Design review of the part built by this model. Coordinates are the model's own, in mm. A direction names the side the tool comes from. Coordinates: 2 decimals unless noted, no trailing zeros. Write each loop counter-clockwise with the first axis right and the second up, starting at its lowest first coordinate (ties: lowest second). Pieces come first, ordered by that corner, then holes. Notation, with made-up numbers: (77.25, 31.25) -> (103.25, 31.25) arc R15 cw to (103.25, 44.25) -> close; hole circle Ø4 at (61, -4.75). An arc over 180 degrees is marked (long way). Write item = value, one per line. Start each with the question number.
Solid Edge part; units mm, degrees
sketch "Sketch1" plane through (0, 0, 0) normal (0, 0, 1) x (1, 0, 0)
  line L0 (58.55, -37.1) -> (-58.55, -37.1)
  line L1 (-58.55, -37.1) -> (-58.55, 37.1)
  line L2 (-58.55, 37.1) -> (58.55, 37.1)
  line L3 (58.55, 37.1) -> (58.55, -37.1)
extrude "Protrusion1" add sketch "Sketch1" against normal blind 2.5
sketch "Sketch2" plane through (0, 0, 0) normal (0, 0, 1) x (1, 0, 0)
  line L0 (56.55, -35.1) -> (-58.55, -35.1)
  line L1 (-58.55, -35.1) -> (-58.55, -37.1)
  line L2 (-58.55, -37.1) -> (58.55, -37.1)
  line L3 (58.55, -37.1) -> (58.55, 37.1)
  line L4 (58.55, 37.1) -> (-58.55, 37.1)
  line L5 (-58.55, 37.1) -> (-58.55, 35.1)
  line L6 (-58.55, 35.1) -> (56.55, 35.1)
  line L7 (56.55, 35.1) -> (56.55, -35.1)
extrude "ExtrudedProtrusion_2" add sketch "Sketch2" along normal blind 7.5
sketch "Sketch3" plane through (0, 0, -2.5) normal (0, 0, -1) x (-1, 0, 0)
  line L0 (-49.1714, -41.0286) -> (-46.45, -35)
  line L1 (-56.45, -35) -> (-46.45, -35)
  line L2 (-56.45, -35) -> (-53.7286, -41.0286)
  arc A0 (-53.7286, -41.0286) -> (-49.1714, -41.0286) centre (-51.45, -40) ccw
  circle A1 centre (-51.45, -40) radius 1.75
  circle A2 centre (53.55, 40) radius 1.75
  line L3 (58.55, 35) -> (55.8286, 41.0286)
  arc A3 (55.8286, 41.0286) -> (51.2714, 41.0286) centre (53.55, 40) ccw
  line L4 (51.2714, 41.0286) -> (48.55, 35)
  line L5 (48.55, 35) -> (58.55, 35)
extrude "Protrusion2" add sketch "Sketch3" against normal up to vertex (15.5 mm away)
fillet "Round_1" radius 1.5 9 edges at (58.55, -37.1, 2.5) (58.55, 37.1, 2.5) (58.55, 0, -2.5) (4.526, 37.1, -2.5) (-5.576, -37.1, -2.5) (57.026, -37.1, -2.5) (-58.55, 0, -2.5) (-58.55, 37.1, 2.5) (-58.55, -37.1, 2.5)
(1) Mouldability with a two-part tool opening along X and no side actions: class faces 1 (the face through (3, 35.1, 4)), 2 (the face through (51.5, -42.5, 5.1)), 3 (the face through (52, -35, 6)) as pulls with the +X half, pulls with the -X half, needs draft (parallel to the pull), parting line crosses it, or undercut.
(2) For line 1 (Y direction, x = 51.45, z = 6.5); line 2 (Y direction, x = -53.55, z = 3.25); line 3 (Y direction, x = 51.45, z = 8.25), list the stretches that pass through material, from the lowest coordinate up.
(3) For faces 4 (the face through (-5, -35.1, 4)), 5 (the face through (1, 1, -2.5)), 6 (the face through (52.84, -41.06, 5.14)), 7 (the face through (3, 37.1, 3)), 8 (the face through (-56.906, 38.642, 5.142)), list the 3-axis set-ups (+Z, -Z, +X, -X, +Y, -Y) from which the entire face can be reached by the end or side of a thin tool; tool diameter is ignored.
(4) Take a section at B-B, the plane x = -53.55. State the section outline as (y, z) points, then the cut area to 3 significant figures.
(5) Take a section at C-C, the plane x = -18. State the section outline as (y, z) points.
(6) Take a section at D-D, the plane y = 23.5. State the section outline as (x, z) points, then the cut area to 3 significant figures.
(7) Take a section at A-A, the plane z = 11. State the section outline as (x, y) points, then the cut area to 3 significant figures.
(8) For pin 1 Ø1 at (x, z) = (-42.5, 1.5) entering from -Y; pin 2 Ø4 at (x, z) = (-22.5, 4.5) entering from +Y; pin 3 Ø10 at (x, y) = (-43, 1) entering from +Z, all flat-tipped, find the tip position at first contact; note any pin that passes through.
Report:
q1.face_1 = undercut
q1.face_2 = parting line crosses it
q1.face_3 = needs draft
q2.line_1 = -42.5 to -41.75, -38.25 to -35, 35.1 to 37.1
q2.line_2 = -37.1 to -35.1, 35 to 38.25, 41.75 to 42.5
q2.line_3 = -42.5 to -41.75, -38.25 to -35
q3.face_4 = +Z, -X
q3.face_5 = -Z, +X, -X, +Y, -Y
q3.face_6 = +Z, -Z
q3.face_7 = +Z, -Z, +X, +Y
q3.face_8 = +Z, -X, +Y
q4.outline = (-37.1, -1) arc R1.5 ccw to (-35.6, -2.5) -> (38.25, -2.5) -> (38.25, 13) -> (35, 13) -> (35, 0) -> (-35.1, 0) -> (-35.1, 7.5) -> (-37.1, 7.5) -> close; (41.75, -2.5) -> (42.5, -2.5) -> (42.5, 13) -> (41.75, 13) -> close
q4.area = 257 mm2
q5.outline = (-37.1, -1) arc R1.5 ccw to (-35.6, -2.5) -> (35.6, -2.5) arc R1.5 ccw to (37.1, -1) -> (37.1, 7.5) -> (35.1, 7.5) -> (35.1, 0) -> (-35.1, 0) -> (-35.1, 7.5) -> (-37.1, 7.5) -> close
q6.outline = (-58.55, -1) arc R1.5 ccw to (-57.05, -2.5) -> (57.05, -2.5) arc R1.5 ccw to (58.55, -1) -> (58.55, 7.5) -> (56.55, 7.5) -> (56.55, 0) -> (-58.55, 0) -> close
q6.area = 307 mm2
q7.outline = (-58.55, 35) -> (-48.55, 35) -> (-51.27, 41.03) arc R2.5 ccw to (-55.83, 41.03) -> close; (46.45, -35) -> (49.17, -41.03) arc R2.5 ccw to (53.73, -41.03) -> (56.45, -35) -> close; hole circle Ø3.5 at (-53.55, 40); hole circle Ø3.5 at (51.45, -40)
q7.area = 78.2 mm2
q8.pin_1 = -37.1
q8.pin_2 = 37.1
q8.pin_3 = 0
